Design review of the part built by this model. Coordinates are the model's own, in mm. A direction names the side the tool comes from. Coordinates: 2 decimals unless noted, no trailing zeros. Write each loop counter-clockwise with the first axis right and the second up, starting at its lowest first coordinate (ties: lowest second). Pieces come first, ordered by that corner, then holes. Notation, with made-up numbers: (81, 38) - (91, 38) arc R33 ccw to (91, 74) - close; hole circle Ø2 at (32.5, 21.25). An arc over 180 degrees is marked (long way). Use a Markdown table: item, result.
from build123d import *

# Parameters (mm, degrees)
CLEVIS_BODY_EXTRUDE1_DEPTH       = 18
SKETCH2_R                        = 6
PIN_HOLES_CUT_EXTRUDE1_DEPTH     = 18
SKETCH3_R                        = 7.5
THREADED_HOLE_CUT_EXTRUDE2_DEPTH = 25
SKETCH5_W                        = 38
SKETCH5_H                        = 18
CLEVIS_GAP_CUT_EXTRUDE4_DEPTH    = 37
FILLET2_R                        = 1.5
CHAMFER2_SIZE                    = 0.5


with BuildPart() as part:
    # Sketch1 → Clevis Body Extrude1 (new body, symmetric)
    with BuildSketch(Plane.XY):
        with BuildLine():
            Line((0, 0), (52, 0))
            ThreePointArc((52, 0), (70, 18), (52, 36))
            Line((52, 36), (0, 36))
            Line((0, 36), (0, 0))
        make_face()
    extrude(amount=CLEVIS_BODY_EXTRUDE1_DEPTH, both=True)

    # Sketch2 → Pin Holes Cut-Extrude1 (cut, symmetric)
    with BuildSketch(Plane.XY):
        with Locations((52, 18)):
            Circle(SKETCH2_R)
    extrude(amount=PIN_HOLES_CUT_EXTRUDE1_DEPTH, both=True, mode=Mode.SUBTRACT)

    # Sketch3 → Threaded Hole Cut-Extrude2 (cut)
    with BuildSketch(Plane.ZY):
        with Locations((0, 18)):
            Circle(SKETCH3_R)
    extrude(amount=-THREADED_HOLE_CUT_EXTRUDE2_DEPTH, mode=Mode.SUBTRACT)

    # Sketch5 → Clevis Gap Cut-Extrude4 (cut, through all)
    with BuildSketch(Plane(origin=(0, 0, 0), x_dir=(1, 0, 0), z_dir=(0, 1, 0))):
        with Locations((53, 0)):
            Rectangle(SKETCH5_W, SKETCH5_H)
    extrude(amount=CLEVIS_GAP_CUT_EXTRUDE4_DEPTH, mode=Mode.SUBTRACT)

    # Fillet2
    fillet2_edges = [part.edges().sort_by_distance(p)[0] for p in [
        (34, 18, 9),
        (34, 18, -9),
    ]]
    fillet(fillet2_edges, radius=FILLET2_R)

    # Chamfer2
    chamfer2_edges = [part.edges().sort_by_distance(p)[0] for p in [
        (0, 18, -7.5),
    ]]
    chamfer(chamfer2_edges, length=CHAMFER2_SIZE)


solid = part.part
(1) Draft analysis for pull direction Y (two halves, no side actions). For faces 4 (the cylindrical face through (12.578, 25.436, -0.976)), 5 (the flat face through (45, 18, 9)), 6 (the flat face through (21, 36, 0)), 7 (the flat face through (20, 0, 0)), state which applies: +Y half, -Y half, draft (parallel to the pull), parting line (faces both ways), or undercut.
Determined:
| item | result |
|---|---|
| face 4 | undercut |
| face 5 | draft |
| face 6 | +Y half |
| face 7 | -Y half |
(2) Take a section at B-B on y = 18. Write out the cut boundary in (x, z).
Determined:
| item | result |
|---|---|
| outline | (0, -18) - (46, -18) - (46, -9) - (35.5, -9) arc R1.5 cw to (34, -7.5) - (34, 7.5) arc R1.5 cw to (35.5, 9) - (46, 9) - (46, 18) - (0, 18) - (0, 8) - (0.5, 7.5) - (25, 7.5) - (25, -7.5) - (0.5, -7.5) - (0, -8) - close; (58, -18) - (70, -18) - (70, -9) - (58, -9) - close; (58, 9) - (70, 9) - (70, 18) - (58, 18) - close |
(3) Machinability: for faces 1 (the flat face through (34, 18, 0)), 2 (the cylindrical face through (46, 18, 14)), 3 (the flat face through (25, 18, 0)), which of the approach directions +Z, -Z, +X, -X, +Y, -Y give a long, thin tool a straight path to every point of the face, cutting with its end or side? Answer none if there is none.
Determined:
| item | result |
|---|---|
| face 1 | +X, +Y, -Y |
| face 2 | +Z, -Z |
| face 3 | -X |
(4) For L1, parallel to Y at x = 52, z = -11; L2, parallel to Z at x = 55, y = 4; L3, parallel to Y at x = 11.75, z = 0, list the stretches that pass through material, from the lowest coordinate up. Write a range as from..to.
Determined:
| item | result |
|---|---|
| L1 | 0..12, 24..36 |
| L2 | -18..-9, 9..18 |
| L3 | 0..10.5, 25.5..36 |
(5) Take a section at A-A on x = 42.5. Write out the cut boundary in (y, z).
Determined:
| item | result |
|---|---|
| outline | (0, -18) - (36, -18) - (36, -9) - (0, -9) - close; (0, 9) - (36, 9) - (36, 18) - (0, 18) - close |
(6) Take a section at C-C on z = 0. Write out the cut boundary in (x, y), and give its area (3 significant figures).
Determined:
| item | result |
|---|---|
| outline | (0, 0) - (34, 0) - (34, 36) - (0, 36) - (0, 26) - (0.5, 25.5) - (25, 25.5) - (25, 10.5) - (0.5, 10.5) - (0, 10) - close |
| area | 849 mm2 |
(7) Take a section at D-D on x = 57. Write out the cut boundary in (y, z), and give its area (3 significant figures).
Determined:
| item | result |
|---|---|
| outline | (0.71, -18) - (14.68, -18) - (14.68, -9) - (0.71, -9) - close; (0.71, 9) - (14.68, 9) - (14.68, 18) - (0.71, 18) - close; (21.32, -18) - (35.29, -18) - (35.29, -9) - (21.32, -9) - close; (21.32, 9) - (35.29, 9) - (35.29, 18) - (21.32, 18) - close |
| area | 503 mm2 |
(8) For pin 1 (3 mm diameter, centred on y = 10.5, z = 11.5, fed in from -X); pin 2 (9 mm diameter, centred on y = 18, z = 0, fed in from +X); pin 3 (7.5 mm diameter, centred on y = 19.5, z = 2, fed in from -X), all flat-tipped, find the tip position at first contact; note any pin that passes through.
Determined:
| item | result |
|---|---|
| pin 1 | x = 0 |
| pin 2 | x = 34 |
| pin 3 | x = 25 |
